from build123d import *

# Parameters (mm, degrees)
F0_R     = 19.1692141119
F1_DEPTH = 12.7
F2_R     = 5.08
F4_R     = 33.249521813
F5_DEPTH = 12.7
F6_R     = 5.08


with BuildPart() as f1:
    # F0 (on Front) → F1 (new body)
    with BuildSketch(Plane.XZ):
        with Locations((-138.7361735106, 32.7932424843)):
            Circle(F0_R)
    extrude(amount=F1_DEPTH)

    # F2
    f2_edges = [f1.edges().sort_by_distance(p)[0] for p in [
        (-157.905388, -12.7, 32.793242),
        (-157.905388, 0, 32.793242),
    ]]
    fillet(f2_edges, radius=F2_R)


with BuildPart() as f5:
    # F4 (on Front) → F5 (new body)
    with BuildSketch(Plane.XZ):
        with Locations((-43.3901064098, 44.0216623247)):
            Circle(F4_R)
    extrude(amount=F5_DEPTH)

    # F6
    f6_edges = [f5.edges().sort_by_distance(p)[0] for p in [
        (-76.639628, 0, 44.021662),
        (-76.639628, -12.7, 44.021662),
    ]]
    fillet(f6_edges, radius=F6_R)


solid = f5.part
Could you check a few things on this model? Use its own coordinates, in mm. Give positions to 0.01 mm unless a question says otherwise; leave off trailing zeros. Order: outer loops, then holes, each group sorted by start corner. A loop starts at its lowest first (then second) coordinate and runs counter-clockwise, first axis right, second up.
1. Suppose I cut it at A-A (y = -11.25). Write out the boundary of the cut face in (x, z), plus the area to 3 significant figures.
Answers below:
outline: circle Ø63.45 at (-43.39, 44.02)
area: 3,160 mm2
2. I need wall thicknesses on L1, parallel to Z at x = -42.5, y = -7.25; L2, parallel to X at y = -5.75, z = 44.5; L3, parallel to Y at x = -20.5, z = 27. Which ranges of each line are inside material? Lowest first, please.
Answers below:
L1: z = 10.78 to 77.26
L2: x = -76.64 to -10.14
L3: y = -12.69 to -0.01
3. For pin 1 (1.5 mm diameter, centred on x = -21, y = -4.5, fed in from +Z); pin 2 (5 mm diameter, centred on x = -45, y = -7.5, fed in from -Z); pin 3 (5 mm diameter, centred on y = -7.5, z = 58, fed in from -X), each with a flat end and sliding along its axis, tell me the tip position at first contact or that it passes through.
Answers below:
pin 1: stops at z = 69.23
pin 2: stops at z = 10.77
pin 3: stops at x = -74.6
4. Suppose I cut it at B-B (y = -2). Write out the boundary of the cut face in (x, z), plus the area to 3 significant figures.
Answers below:
outline: circle Ø64.42 at (-43.39, 44.02)
area: 3,260 mm2
